For this review, take the finished solid that the model builds, in its own axes (mm). A direction names the side the tool comes from. Coordinates: 2 decimals unless noted, no trailing zeros. Write each loop counter-clockwise with the first axis right and the second up, starting at its lowest first coordinate (ties: lowest second). Pieces come first, ordered by that corner, then holes.
```python
from build123d import *

# Parameters (mm, degrees)
SKETCH2_R          = 4.064
CUT_EXTRUDE1_DEPTH = 8.382
CUT_EXTRUDE3_START = -15.24
CUT_EXTRUDE3_DEPTH = 15.24
FILLET2_R          = 0.508


with BuildPart() as part:
    # Sketch1 → Revolve1 (revolve)
    with BuildSketch(Plane(origin=(0, 0, 0), x_dir=(0, 0, -1), z_dir=(1, 0, 0))):
        Polygon((0, 0), (4.064, 0), (4.064, 13.97), (4.064, 29.21), (6.35, 29.21), (6.35, 39.37), (0, 39.37), align=None)
    revolve(axis=Axis((0, 0, 0), (0, 1, 0)))

    # Sketch2 → Cut-Extrude1 (cut)
    with BuildSketch(Plane(origin=(0, 39.37, 0), x_dir=(1, 0, 0), z_dir=(0, 1, 0))):
        with Locations(Location((0, 0, 0), (0, 0, 90))):
            Circle(SKETCH2_R)
    extrude(amount=-CUT_EXTRUDE1_DEPTH, mode=Mode.SUBTRACT)

    # Sketch3 → Cut-Extrude3 (cut)
    with BuildSketch(Plane.XZ.offset(CUT_EXTRUDE3_START)):
        with BuildLine():
            Line((-2.032, 3.519527241), (2.032, 3.519527241))
            ThreePointArc((2.032, 3.519527241), (0, 4.064), (-2.032, 3.519527241))
        make_face()
        with BuildLine():
            ThreePointArc((4.064, 0), (3.519527241, 2.032), (2.032, 3.519527241))
            Line((2.032, 3.519527241), (4.064, 0))
        make_face()
        with BuildLine():
            ThreePointArc((2.032, -3.519527241), (3.519527241, -2.032), (4.064, 0))
            Line((4.064, 0), (2.032, -3.519527241))
        make_face()
        with BuildLine():
            ThreePointArc((-2.032, -3.519527241), (0, -4.064), (2.032, -3.519527241))
            Line((2.032, -3.519527241), (-2.032, -3.519527241))
        make_face()
        with BuildLine():
            Line((-2.032, -3.519527241), (-4.064, 0))
            ThreePointArc((-4.064, 0), (-3.519527241, -2.032), (-2.032, -3.519527241))
        make_face()
        with BuildLine():
            Line((-4.064, 0), (-2.032, 3.519527241))
            ThreePointArc((-2.032, 3.519527241), (-3.519527241, 2.032), (-4.064, 0))
        make_face()
    extrude(amount=CUT_EXTRUDE3_DEPTH, mode=Mode.SUBTRACT)

    # Fillet2
    fillet2_edges = [part.edges().sort_by_distance(p)[0] for p in [
        (-4.064, 7.62, 0),
        (2.032, 7.62, -3.519527241),
        (2.032, 7.62, 3.519527241),
        (-2.032, 7.62, 3.519527241),
        (4.064, 7.62, 0),
        (-2.032, 7.62, -3.519527241),
    ]]
    fillet(fillet2_edges, radius=FILLET2_R)


solid = part.part
```
Q1. For probe 1 along X at (y, z) = (36.25, 0); probe 2 along Y at (x, z) = (-2.25, 2.75); probe 3 along Y at (x, z) = (-0.25, -4.75), list the stretches that pass through material, from the lowest coordinate up.
Ans:
probe 1: x = -6.35 to -4.06, 4.06 to 6.35
probe 2: y = 0 to 30.99
probe 3: y = 29.21 to 39.37
Q2. Add section A-A (x = 0). State the section outline as (y, z) points, then the cut area to 3 significant figures.
Ans:
outline: (0, -3.52) - (15.24, -3.52) - (15.24, -4.06) - (29.21, -4.06) - (29.21, -6.35) - (39.37, -6.35) - (39.37, -4.06) - (30.99, -4.06) - (30.99, 4.06) - (39.37, 4.06) - (39.37, 6.35) - (29.21, 6.35) - (29.21, 4.06) - (15.24, 4.06) - (15.24, 3.52) - (0, 3.52) - close
area: 282 mm2
Q3. Add section D-D (x = 3). State the section outline as (y, z) points, then the cut area to 3 significant figures.
Ans:
outline: (0, -1.84) - (15.24, -1.84) - (15.24, -2.74) - (29.21, -2.74) - (29.21, -5.6) - (39.37, -5.6) - (39.37, -2.74) - (30.99, -2.74) - (30.99, 2.74) - (39.37, 2.74) - (39.37, 5.6) - (29.21, 5.6) - (29.21, 2.74) - (15.24, 2.74) - (15.24, 1.84) - (0, 1.84) - close
area: 201 mm2
Q4. Draft analysis for pull direction Z (two halves, no side actions). For faces 1 (the flat face through (3.036, 7.727, 1.781)), 2 (the cylindrical face through (6.2, 34.36, 1.38)), 3 (the cylindrical face through (3.967, 35.238, 0.881)), state which applies: +Z half, -Z half, draft (parallel to the pull), parting line (faces both ways), or undercut.
Ans:
face 1: +Z half
face 2: parting line
face 3: undercut
Q5. Clearance check with flat-ended pins moving along their axes: pin 1 Ø3 at (x, y) = (-0.5, 6.5) entering from +Z; pin 2 Ø2 at (y, z) = (13, 0) entering from -X; pin 3 Ø4 at (x, z) = (-1, -1.5) entering from -Y; pin 4 Ø3 at (x, y) = (-0.5, 4.5) entering from -Z. State where each tip first meets the part, or that it passes through.
Ans:
pin 1: stops at z = 3.52
pin 2: stops at x = -3.99
pin 3: stops at y = 0
pin 4: stops at z = -3.52
Q6. Add section C-C (y = 17). State the section outline as (x, z) points.
Ans:
outline: circle Ø8.13 at (0, 0)
Q7. Tool access review of faces 4 (the flat face through (4.1, 29.21, 1.3)), 5 (the flat face through (3.06, 7.73, -1.74)), 6 (the flat face through (-3.06, 7.73, 1.74)), 7 (the flat face through (0, 30.988, 0)): name each direction out of +Z, -Z, +X, -X, +Y, -Y from which nothing blocks a thin tool from reaching the whole face with its end or side.
Ans:
face 4: -Y
face 5: -Z, +X, -Y
face 6: +Z, -X, -Y
face 7: +Y
Q8. Add section B-B (y = 7). State the section outline as (x, z) points, then the cut area to 3 significant figures.
Ans:
outline: (-3.92, -0.25) - (-2.18, -3.27) arc R0.51 ccw to (-1.74, -3.52) - (1.74, -3.52) arc R0.51 ccw to (2.18, -3.27) - (3.92, -0.25) arc R0.51 ccw to (3.92, 0.25) - (2.18, 3.27) arc R0.51 ccw to (1.74, 3.52) - (-1.74, 3.52) arc R0.51 ccw to (-2.18, 3.27) - (-3.92, 0.25) arc R0.51 ccw to start
area: 42.8 mm2
